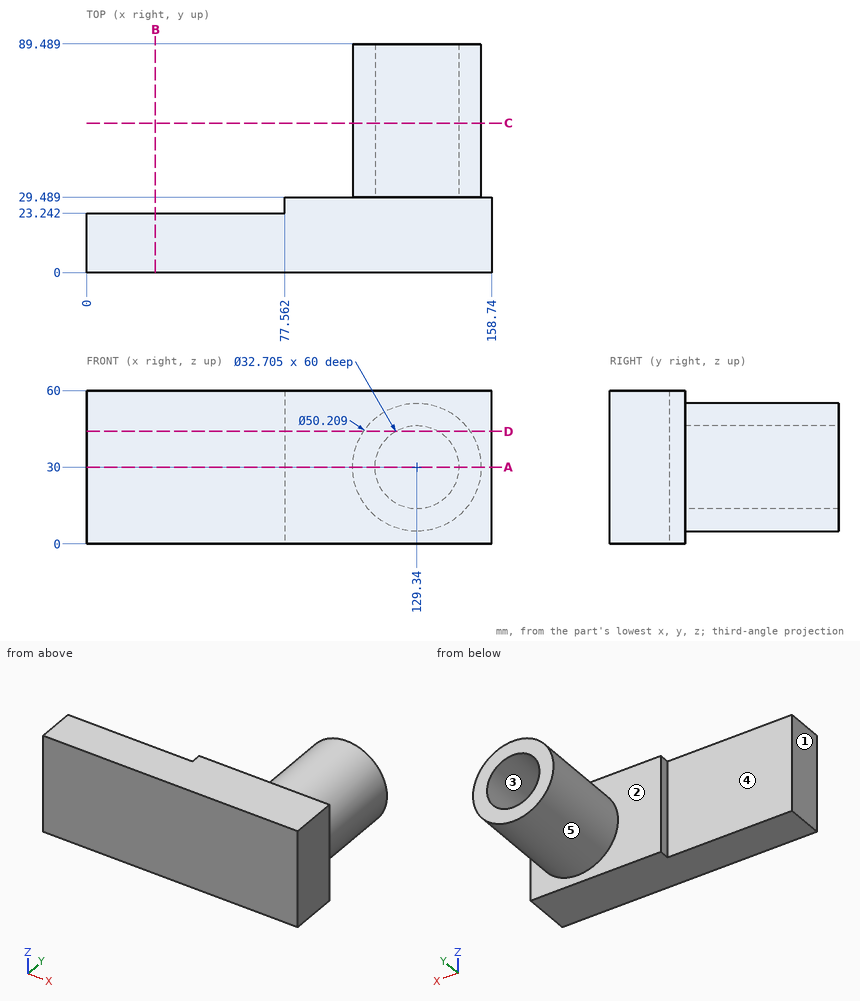
Part print with two shaded views. Sizes in mm from the minimum x, y, z corner. A direction names the side the tool comes from. Round coordinates to 2 decimals unless told otherwise and drop trailing zeros. Order: outer loops, then holes, each group sorted by start corner. A loop starts at its lowest first (then second) coordinate and runs counter-clockwise, first axis right, second up. Notation, with made-up numbers: (88.5, -33.5) - (131.5, -33.5) arc R11 cw to (131.5, -25.5) - close; hole circle Ø10 at (-16.5, 56). An arc over 180 degrees is marked (long way). Answer as CSV lines item,"result". Start each with the question number.
1. Drill centre lines: L1, parallel to X at y = 54, z = 30 (1 decimal); L2, parallel to Y at x = 50.5, z = 26.5; L3, parallel to Y at x = 95, z = 27.5. Where is each one in solid material? Low to high. Write a range as [from, to].
2. Saw through at B-B, the plane x = 27. Write the cut outline in (y, z), and give its area (3 significant figures).
3. Tool access for the marked faces 1 and 2: list every direction of +Z, -Z, +X, -X, +Y, -Y with a clear straight run to the whole face (end or side of a thin tool).
4. Saw through at D-D, the plane z = 44. Write the cut outline in (x, y), and give its area (3 significant figures).
5. Pin check, flat tips, straight feed: pin 1 (2 mm diameter, centred on x = 92.5, z = 50.5, fed in from +Y); pin 2 (5 mm diameter, centred on y = 27, z = 19.5, fed in from -X); pin 3 (10 mm diameter, centred on y = 57, z = 31, fed in from -X). Stop position of each tip, or through.
6. Saw through at C-C, the plane y = 58.5. Write the cut outline in (x, z) (1 decimal).
7. Saw through at A-A, the plane z = 30. Write the cut outline in (x, y) (1 decimal).
8. Pull direction Z, two halves, no side cores. Call the marked faces 3, 4 and 5: +Z half, -Z half, draft (parallel to the pull), parting line (faces both ways), or undercut.
Model answer:
1,L1,"x = [104.2, 113], [145.7, 154.4]"
1,L2,"y = [0, 23.24]"
1,L3,"y = [0, 29.49]"
2,outline,"(0, 0) - (23.24, 0) - (23.24, 60) - (0, 60) - close"
2,area,"1,390 mm²"
3,face 1,"+Z, -Z, -X, +Y, -Y"
3,face 2,"+Y"
4,outline,"(0, 0) - (158.74, 0) - (158.74, 29.49) - (150.18, 29.49) - (150.18, 89.49) - (137.79, 89.49) - (137.79, 29.49) - (120.89, 29.49) - (120.89, 89.49) - (108.5, 89.49) - (108.5, 29.49) - (77.56, 29.49) - (77.56, 23.24) - (0, 23.24) - close"
4,area,"5,680 mm²"
5,pin 1,"stops at y = 29.49"
5,pin 2,"stops at x = 77.56"
5,pin 3,"stops at x = 104.24"
6,outline,"circle Ø50.2 at (129.3, 30); hole circle Ø32.7 at (129.3, 30)"
7,outline,"(0, 0) - (158.7, 0) - (158.7, 29.5) - (154.4, 29.5) - (154.4, 89.5) - (145.7, 89.5) - (145.7, 29.5) - (113, 29.5) - (113, 89.5) - (104.2, 89.5) - (104.2, 29.5) - (77.6, 29.5) - (77.6, 23.2) - (0, 23.2) - close"
8,face 3,"undercut"
8,face 4,"draft"
8,face 5,"parting line"
